Design review of the part built by this model. Coordinates are the model's own, in mm. A direction names the side the tool comes from. Give positions to 0.01 mm unless a question says otherwise; leave off trailing zeros. Write each loop counter-clockwise with the first axis right and the second up, starting at its lowest first coordinate (ties: lowest second). Pieces come first, ordered by that corner, then holes. Notation, with made-up numbers: (12, 32) -> (66, 32) arc R10 ccw to (66, 40) -> close; hole circle Ø10 at (43.5, 25). An arc over 180 degrees is marked (long way). Use CSV: the item, a comma, the result in double quotes.
```python
from build123d import *

# Parameters (mm, degrees)
SKETCH1_R                                       = 57.15
BOSS_EXTRUDE1_DEPTH                             = 6.35
SKETCH2_W                                       = 44.45
SKETCH2_H                                       = 31.75
BOSS_EXTRUDE2_DEPTH                             = 3.81
SKETCH3_W                                       = 13
SKETCH3_H                                       = 19.4
CUT_EXTRUDE1_DEPTH                              = 82.458397971
SKETCH4_W                                       = 39.77
SKETCH4_H                                       = 27.02
CUT_EXTRUDE2_DEPTH                              = 8.66
FILLET1_R                                       = 1.5875
CUT_EXTRUDE3_DEPTH                              = 1.5875
CBORE_FOR_6_PAN_HEAD_MACHINE_SCREW1_D           = 3.7973
CBORE_FOR_6_PAN_HEAD_MACHINE_SCREW1_CBORE_D     = 7.54126
CBORE_FOR_6_PAN_HEAD_MACHINE_SCREW1_CBORE_DEPTH = 2.4638
CIRPATTERN1_COUNT                               = 6
SKETCH27_R                                      = 63.5
SKETCH27_R_2                                    = 48.133
CUT_EXTRUDE14_DEPTH                             = 82.071372876
CUT_EXTRUDE15_DEPTH                             = 2.54


with BuildPart() as part:
    # Sketch1 → Boss-Extrude1 (new body)
    with BuildSketch(Plane.XY):
        Circle(SKETCH1_R)
    extrude(amount=BOSS_EXTRUDE1_DEPTH)

    # Sketch2 → Boss-Extrude2 (add)
    with BuildSketch(Plane.XY.offset(6.35)):
        with Locations((0, 29.80529526)):
            Rectangle(SKETCH2_W, SKETCH2_H)
    extrude(amount=BOSS_EXTRUDE2_DEPTH)

    # Sketch3 → Cut-Extrude1 (cut, through all)
    with BuildSketch(Plane.XY.offset(10.16)):
        with Locations((-9.575, 29.80529526)):
            Rectangle(SKETCH3_W, SKETCH3_H)
        with Locations((9.575, 29.80529526)):
            Rectangle(SKETCH3_W, SKETCH3_H)
    extrude(amount=-CUT_EXTRUDE1_DEPTH, mode=Mode.SUBTRACT)

    # Sketch4 → Cut-Extrude2 (cut)
    with BuildSketch(Plane(origin=(0, 0, 0), x_dir=(-1, 0, 0), z_dir=(0, 0, -1))):
        with Locations((0, 29.80529526)):
            Rectangle(SKETCH4_W, SKETCH4_H)
    extrude(amount=-CUT_EXTRUDE2_DEPTH, mode=Mode.SUBTRACT)

    # Fillet1
    fillet1_edges = [part.edges().sort_by_distance(p)[0] for p in [
        (-19.885, 16.29529526, 4.33),
        (-19.885, 43.31529526, 4.33),
        (19.885, 43.31529526, 4.33),
        (19.885, 16.29529526, 4.33),
    ]]
    fillet(fillet1_edges, radius=FILLET1_R)

    # Sketch8 → Cut-Extrude3 (cut)
    with BuildSketch(Plane(origin=(0, 0, 0), x_dir=(-1, 0, 0), z_dir=(0, 0, -1))):
        with BuildLine():
            Line((18.2975, 44.90279526), (-18.2975, 44.90279526))
            ThreePointArc((-18.2975, 44.90279526), (-20.54256403, 43.97285929), (-21.4725, 41.72779526))
            Line((-21.4725, 41.72779526), (-21.4725, 32.98029526))
            ThreePointArc((-21.4725, 32.98029526), (-24.6475, 29.80529526), (-21.4725, 26.63029526))
            Line((-21.4725, 26.63029526), (-21.4725, 17.88279526))
            ThreePointArc((-21.4725, 17.88279526), (-20.54256403, 15.637731229), (-18.2975, 14.70779526))
            Line((-18.2975, 14.70779526), (18.2975, 14.70779526))
            ThreePointArc((18.2975, 14.70779526), (20.54256403, 15.637731229), (21.4725, 17.88279526))
            Line((21.4725, 17.88279526), (21.4725, 26.63029526))
            ThreePointArc((21.4725, 26.63029526), (24.6475, 29.80529526), (21.4725, 32.98029526))
            Line((21.4725, 32.98029526), (21.4725, 41.72779526))
            ThreePointArc((21.4725, 41.72779526), (20.54256403, 43.97285929), (18.2975, 44.90279526))
        make_face()
    extrude(amount=-CUT_EXTRUDE3_DEPTH, mode=Mode.SUBTRACT)

    # CBORE for #6 Pan Head Machine Screw1 (through all)
    with Locations(Plane(origin=(0, 0, 0), x_dir=(-1, 0, 0), z_dir=(0, 0, -1))):
        with Locations((-43.994090512, -25.4)):
            cbore_for_6_pan_head_machine_screw1 = CounterBoreHole(CBORE_FOR_6_PAN_HEAD_MACHINE_SCREW1_D / 2, CBORE_FOR_6_PAN_HEAD_MACHINE_SCREW1_CBORE_D / 2, CBORE_FOR_6_PAN_HEAD_MACHINE_SCREW1_CBORE_DEPTH)

    # CirPattern1: CBORE for #6 Pan Head Machine Screw1 ×6 about axis
    cirpattern1_axis = Axis((0, 0, 0), (0, 0, 1))
    for i in range(1, CIRPATTERN1_COUNT):
        add(cbore_for_6_pan_head_machine_screw1.rotate(cirpattern1_axis, i * 360 / CIRPATTERN1_COUNT), mode=Mode.SUBTRACT)

    # Sketch27 → Cut-Extrude14 (cut, through all)
    with BuildSketch(Plane.XY.offset(6.35)):
        Circle(SKETCH27_R)
        Circle(SKETCH27_R_2, mode=Mode.SUBTRACT)
    extrude(amount=CUT_EXTRUDE14_DEPTH, mode=Mode.SUBTRACT)

    # Sketch28 → Cut-Extrude15 (cut)
    with BuildSketch(Plane(origin=(0, 0, 1.5875), x_dir=(-1, 0, 0), z_dir=(0, 0, -1))):
        with BuildLine():
            Line((-21.4725, 31.39279526), (-19.885, 31.39279526))
            Line((-19.885, 31.39279526), (-19.885, 28.21779526))
            Line((-19.885, 28.21779526), (-21.4725, 28.21779526))
            ThreePointArc((-21.4725, 28.21779526), (-23.06, 29.80529526), (-21.4725, 31.39279526))
        make_face()
        with BuildLine():
            Line((21.4725, 28.21779526), (19.885, 28.21779526))
            Line((19.885, 28.21779526), (19.885, 31.39279526))
            Line((19.885, 31.39279526), (21.4725, 31.39279526))
            ThreePointArc((21.4725, 31.39279526), (23.06, 29.80529526), (21.4725, 28.21779526))
        make_face()
    extrude(amount=-CUT_EXTRUDE15_DEPTH, mode=Mode.SUBTRACT)


solid = part.part
```
(1) Mouldability with a two-part tool opening along Y and no side actions: class faces 4 (the face through (0, 13.93, 8)), 5 (the face through (-57.095, 2.513, 3.131)), 6 (the face through (0, 45.68, 8)), 7 (the face through (-24.647, 29.735, 0.783)) as +Y half, -Y half, draft (parallel to the pull), parting line (faces both ways), or undercut.
Established:
face 4,"-Y half"
face 5,"parting line"
face 6,"+Y half"
face 7,"undercut"
(2) Tool access review of faces 1 (the face through (-0.412, 48.946, 4.434)), 2 (the face through (0, 30, 8.66)), 3 (the face through (-22.225, 28, 8)): name each direction out of +Z, -Z, +X, -X, +Y, -Y from which nothing blocks a thin tool from reaching the whole face with its end or side.
Established:
face 1,"+Z, -Z"
face 2,"-Z"
face 3,"+Z, -X, +Y, -Y"
(3) Take a section at B-B (y = -25.4). Write out the cut boundary in (x, z), then the cut area to 3 significant figures.
Established:
outline,"(-51.2, 0) -> (-47.76, 0) -> (-47.76, 2.46) -> (-45.89, 2.46) -> (-45.89, 6.35) -> (-51.2, 6.35) -> close; (-42.1, 2.46) -> (-40.22, 2.46) -> (-40.22, 0) -> (40.22, 0) -> (40.22, 2.46) -> (42.1, 2.46) -> (42.1, 6.35) -> (-42.1, 6.35) -> close; (45.89, 2.46) -> (47.76, 2.46) -> (47.76, 0) -> (51.2, 0) -> (51.2, 6.35) -> (45.89, 6.35) -> close"
area,"584 mm2"
(4) Take a section at D-D (y = 0). Write out the cut boundary in (x, z).
Established:
outline,"(-57.15, 0) -> (57.15, 0) -> (57.15, 6.35) -> (-57.15, 6.35) -> close"
(5) Clearance check with flat-ended pins moving along their axes: pin 1 (6 mm diameter, centred on x = 0, y = 50.8, fed in from +Z); pin 2 (1.3 mm diameter, centred on y = 20.5, z = 0.5, fed in from +X); pin 3 (1.1 mm diameter, centred on x = -3.5, z = 7.5, fed in from +Y); pin 4 (3 mm diameter, centred on x = -39.5, z = 8, fed in from -Y). State where each tip first meets the part, or that it passes through.
Established:
pin 1,"stops at z = 6.35"
pin 2,"stops at x = 53.59"
pin 3,"stops at y = 45.68"
pin 4,"passes through"
(6) Take a section at C-C (x = -26.5). Write out the cut boundary in (y, z).
Established:
outline,"(-50.63, 0) -> (50.63, 0) -> (50.63, 6.35) -> (-50.63, 6.35) -> close"
(7) Take a section at A-A (y = 50.8). Write out the cut boundary in (x, z), then the cut area to 3 significant figures.
Established:
outline,"(-26.18, 0) -> (-3.77, 0) -> (-3.77, 2.46) -> (-1.9, 2.46) -> (-1.9, 6.35) -> (-26.18, 6.35) -> close; (1.9, 2.46) -> (3.77, 2.46) -> (3.77, 0) -> (26.18, 0) -> (26.18, 6.35) -> (1.9, 6.35) -> close"
area,"299 mm2"
(8) For line 1 along Y through (x, z) = (0, 1); line 2 along X through (y, z) = (-25, 4); line 3 along Z through (x, y) = (12.5, 43.5), list the stretches that pass through material, from the lowest coordinate up. Write a range as [from, to].
Established:
line 1,"y = [-57.15, -54.57], [-47.03, 14.71], [44.9, 47.03], [54.57, 57.15]"
line 2,"x = [-51.39, -45.85], [-42.14, 42.14], [45.85, 51.39]"
line 3,"z = [1.59, 10.16]"
